Check sheet for the modelled part. Datum: model origin and axes. Units: mm. Face numbers are marked on the shaded views. A direction names the side the tool comes from. Round coordinates to 2 decimals unless told otherwise and drop trailing zeros. Write each loop counter-clockwise with the first axis right and the second up, starting at its lowest first coordinate (ties: lowest second). Pieces come first, ordered by that corner, then holes.
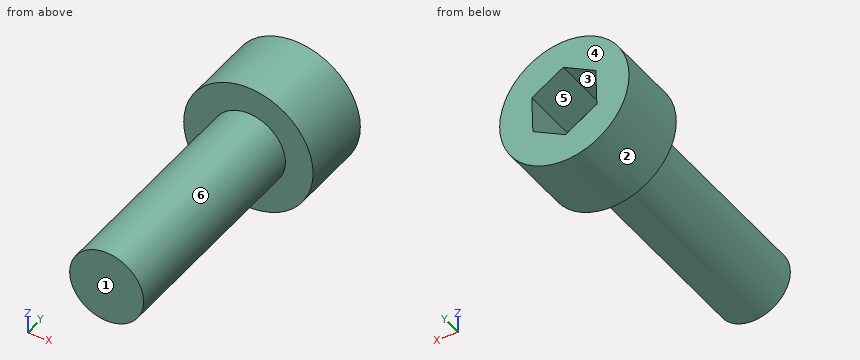
Autodesk Inventor part; units mm, degrees
ref_plane "YZ Plane" through (0, 0, 0) normal (1, 0, 0) x (0, 1, 0)
ref_plane "XZ Plane" through (0, 0, 0) normal (0, 1, 0) x (-1, 0, 0)
ref_plane "XY Plane" through (0, 0, 0) normal (0, 0, 1) x (1, 0, 0)
sketch "Sketch1" plane through (0, 0, 0) normal (0, 1, 0) x (-1, 0, 0)
  circle A0 centre (0, 0) radius 2
  dimension "d0" = 4
extrude "Extrusion1" add sketch "Sketch1" along normal blind 12
sketch "Sketch2" plane through (0, 12, 0) normal (0, 1, 0) x (1, 0, 0)
  circle A0 centre (0, 0) radius 3.5
  dimension "d5" = 7
thread "Thread1"
extrude "Extrusion2" add sketch "Sketch2" along normal blind 4
sketch "Sketch3" plane through (0, 16, 0) normal (0, 1, 0) x (1, 0, 0)
  circle A0 centre (0, 0) radius 3.5
  circle A1 centre (0, 0) radius 2
  line L0 (-1.7603, 0.9494) -> (-0.058, 1.9992)
  line L1 (-0.058, 1.9992) -> (1.7023, 1.0498)
  line L2 (1.7023, 1.0498) -> (1.7603, -0.9494)
  line L3 (1.7603, -0.9494) -> (0.058, -1.9992)
  line L4 (0.058, -1.9992) -> (-1.7023, -1.0498)
  line L5 (-1.7023, -1.0498) -> (-1.7603, 0.9494)
extrude "Extrusion3" cut sketch "Sketch3" against normal blind 3 contours L2 L3 L4 L5 L0 L1
properties part number "M4_12mm" material "Steel, Alloy"
1. Set-up check for the marked faces 4, 5 and 6: record each of +Z, -Z, +X, -X, +Y, -Y from which the full face is reachable in a straight line by a thin tool's end or side.
2. Scan lines: line 1 along Y through (x, z) = (-0.75, 3); line 2 along Y through (x, z) = (-1.25, -0.75); line 3 along X through (y, z) = (13.75, -0.75). Record each from-to range of solid material in increasing order.
3. Sectioned sample at B-B, the plane x = -0.25. Enter the section's corners in (y, z).
4. Release check for a two-part mould opening along X. For the marked faces 1, 2 and 3 record: released by +X, released by -X, zero draft, split by the parting line, or undercut.
5. Sectioned sample at D-D, the plane x = -2.25. Enter the section's corners in (y, z), plus the area to 3 significant figures.
6. Sectioned sample at C-C, the plane y = 11.5. Enter the section's corners in (x, z).
7. Go/stop test with flat-tipped pins: pin 1 (2 mm diameter, centred on x = -2.5, z = -2.5, fed in from -Y); pin 2 (1.1 mm diameter, centred on x = 0.5, z = 0.5, fed in from +Y); pin 3 (1.5 mm diameter, centred on x = 1, z = -0.5, fed in from +Y); pin 4 (1 mm diameter, centred on y = 2, z = -0.5, fed in from +X). Record where each tip stops, or that it passes through.
8. Sectioned sample at A-A, the plane z = -1.75. Enter the section's corners in (x, y).
Computed values:
1. face 4: +Z, -Z, +X, -X, +Y
1. face 5: +Y
1. face 6: -Y
2. line 1: y = 12 to 16
2. line 2: y = 0 to 13
2. line 3: x = -3.42 to -1.75, 1.71 to 3.42
3. outline: (0, -1.98) - (12, -1.98) - (12, -3.49) - (16, -3.49) - (16, -1.88) - (13, -1.88) - (13, 1.83) - (16, 1.83) - (16, 3.49) - (12, 3.49) - (12, 1.98) - (0, 1.98) - close
4. face 1: zero draft
4. face 2: split by the parting line
4. face 3: undercut
5. outline: (12, -2.68) - (16, -2.68) - (16, 2.68) - (12, 2.68) - close
5. area: 21.4 mm2
6. outline: circle Ø4 at (0, 0)
7. pin 1: stops at y = 12
7. pin 2: stops at y = 13
7. pin 3: stops at y = 16
7. pin 4: stops at x = 2
8. outline: (-3.03, 12) - (-0.97, 12) - (-0.97, 0) - (0.97, 0) - (0.97, 12) - (3.03, 12) - (3.03, 16) - (0.4, 16) - (0.4, 13) - (-0.46, 13) - (-0.46, 16) - (-3.03, 16) - close
